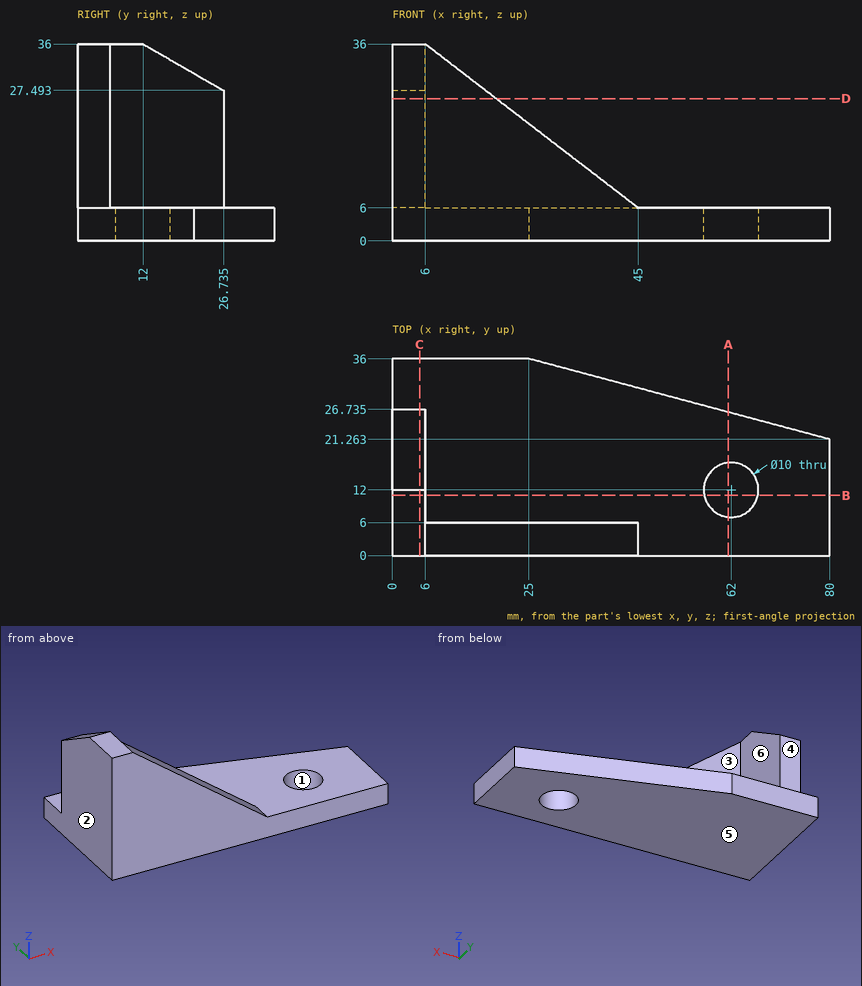
Geometry check sheet. Reference: drawing and pictorial views, mm from the part's lowest x, y, z. A direction names the side the tool comes from. Round coordinates to 2 decimals unless told otherwise and drop trailing zeros. Loops run counter-clockwise (first coordinate to the right, second up) from the corner with the lowest first, then second, coordinate; pieces in that order, holes last. Notation, with made-up numbers: (2.5, 16) - (35.5, 16) arc R25 ccw to (35.5, 38) - close; hole circle Ø5 at (36, 15). An arc over 180 degrees is marked (long way). Write item = value, one per line. Start each with the question number.
Q1. Depth check by flat-ended pin: P1, Ø1.8, axis at x = 3, z = 13.5, coming from the +Y side (3 decimals); P2, Ø4, axis at y = 14, z = 15.5, coming from the +X side; P3, Ø9, axis at x = 27, z = 22.5, coming from the +Y side; P4, Ø6, axis at x = 62, y = 12, coming from the -Z side. Enter the tip coordinate at first touch or a pass-through.
Q2. Section check D-D (z = 26). Record the boundary of the cut face in (x, y) (1 decimal).
Q3. Section check B-B (y = 11). Record the boundary of the cut face in (x, z).
Q4. Thickness scan on L1, parallel to Z at x = 32, y = 32. Record the ranges inside material, lowest first.
Q5. Section check A-A (x = 61.5). Record the boundary of the cut face in (y, z) (1 decimal), plus the area to 3 significant figures.
Q6. Section check C-C (x = 5). Record the boundary of the cut face in (y, z) (1 decimal), plus the area to 3 significant figures.
Q7. Access from +Z, -Z, +X, -X, +Y, -Y to the whole of each face (thin tool, end or side, straight path). Record for the marked faces 4, 5 and 6.
Q8. Release check for a two-part mould opening along X. For the marked faces 1, 2 and 3 record: pulls with the +X half, pulls with the -X half, needs draft (parallel to the pull), parting line crosses it, or undercut.
Derived:
q1.P1 = 26.735
q1.P2 = 6
q1.P3 = 6
q1.P4 = through
q2.outline = (0, 0) - (19, 0) - (19, 6) - (6, 6) - (6, 26.7) - (0, 26.7) - close
q3.outline = (0, 0) - (57.1, 0) - (57.1, 6) - (6, 6) - (6, 36) - (0, 36) - close; (66.9, 0) - (80, 0) - (80, 6) - (66.9, 6) - close
q4.L1 = 0 to 6
q5.outline = (0, 0) - (7, 0) - (7, 6) - (0, 6) - close; (17, 0) - (26.2, 0) - (26.2, 6) - (17, 6) - close
q5.area = 97.6 mm^2
q6.outline = (0, 0) - (36, 0) - (36, 6) - (26.7, 6) - (26.7, 27.5) - (12, 36) - (0, 36) - close
q6.area = 955 mm^2
q7.face_4 = +Z, +X, -X, +Y
q7.face_5 = -Z, +X, -X, +Y, -Y
q7.face_6 = +Z, +X, +Y
q8.face_1 = undercut
q8.face_2 = pulls with the -X half
q8.face_3 = needs draft
